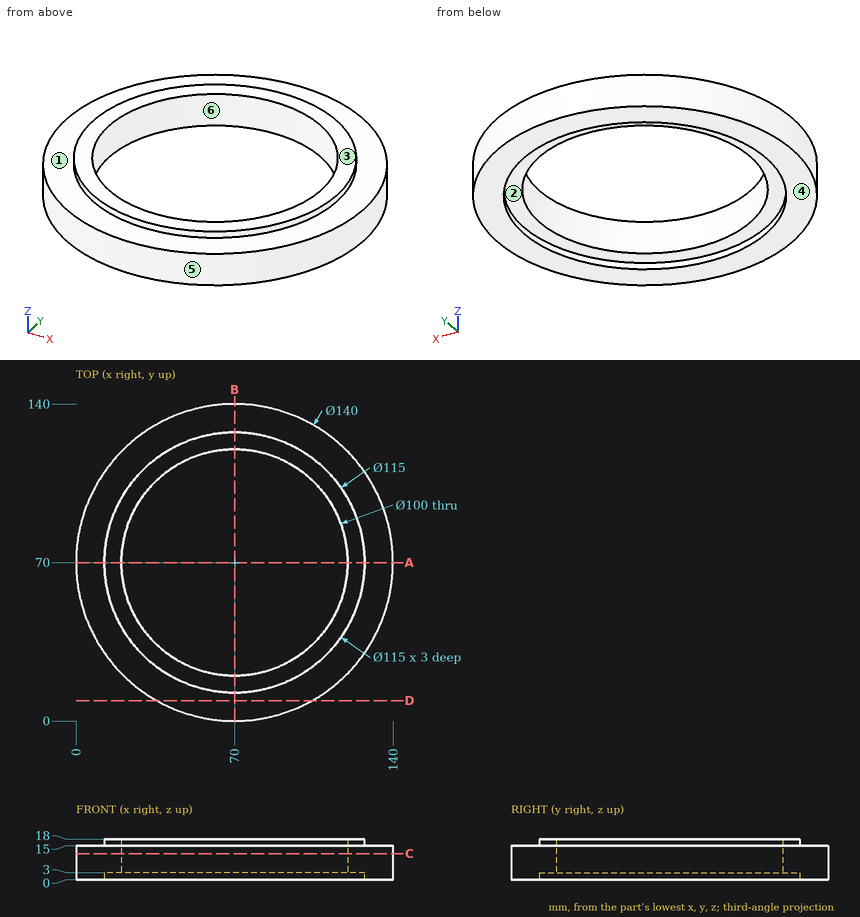
Geometry: see drawing. Coordinates: mm, zero at the bounding-box minimum. A direction names the side the tool comes from. Round coordinates to 2 decimals unless told otherwise and drop trailing zeros. Write each loop counter-clockwise with the first axis right and the second up, starting at its lowest first coordinate (ties: lowest second). Pieces come first, ordered by that corner, then holes.
Item 1: Mould query, pull axis X, two halves, no side actions, for the marked faces 4, 5 and 6. Classes: +X half, -X half, draft (parallel to the pull), parting line (faces both ways), or undercut.
Item 2: Pin query (flat end, axial travel): P1, Ø3, axis at x = 25.5, z = 6.5, coming from the -Y side; P2, Ø1.5, axis at y = 126, z = 6, coming from the +X side; P3, Ø2, axis at x = 53, z = 12.5, coming from the -Y side. Return the tip coordinate at first contact, or that it passes through.
Item 3: Section query A-A (y = 70). Return loops of the section in (x, z).
Item 4: Section query C-C (z = 11.5). Return loops of the section in (x, y), plus the area to 3 significant figures.
Item 5: Set-up query: the marked faces 1, 2 and 3. Return all of +Z, -Z, +X, -X, +Y, -Y with unobstructed straight access to the full face (end or side cutting, diameter ignored); none if empty.
Item 6: Material intervals for L1, parallel to Y at x = 70, z = 0.9; L2, parallel to Z at x = 66, y = 123.5; L3, parallel to Y at x = 96, z = 2, sorted ascending.
Item 7: Section query D-D (y = 9). Return loops of the section in (x, z), plus the area to 3 significant figures.
Completed:
1. face 4: draft
1. face 5: parting line
1. face 6: undercut
2. P1: stops at y = 14.76
2. P2: stops at x = 112.98
2. P3: stops at y = 1.85
3. outline: (0, 0) - (12.5, 0) - (12.5, 3) - (20, 3) - (20, 18) - (12.5, 18) - (12.5, 15) - (0, 15) - close; (120, 3) - (127.5, 3) - (127.5, 0) - (140, 0) - (140, 15) - (127.5, 15) - (127.5, 18) - (120, 18) - close
4. outline: circle Ø140 at (70, 70); hole circle Ø100 at (70, 70)
4. area: 7,540 mm2
5. face 1: +Z
5. face 2: -Z
5. face 3: +Z, +X, -X, +Y, -Y
6. L1: y = 0 to 12.5, 127.5 to 140
6. L2: z = 3 to 18
6. L3: y = 5.01 to 18.71, 121.29 to 134.99
7. outline: (35.66, 0) - (104.34, 0) - (104.34, 15) - (35.66, 15) - close
7. area: 1,030 mm2
